Here's the drawing with two shaded views (mm, measured from the low corner). I have some questions. A direction names the side the tool comes from. Round coordinates to 2 decimals unless told otherwise and drop trailing zeros. Write each loop counter-clockwise with the first axis right and the second up, starting at its lowest first coordinate (ties: lowest second). Pieces come first, ordered by that corner, then holes. Notation, with made-up numbers: (55.5, -20) - (67.5, -20) arc R21 ccw to (67.5, 2) - close; hole circle Ø2 at (26.25, 35). An arc over 180 degrees is marked (long way). Return JSON: item names as keys, results as strings. Group by question number.
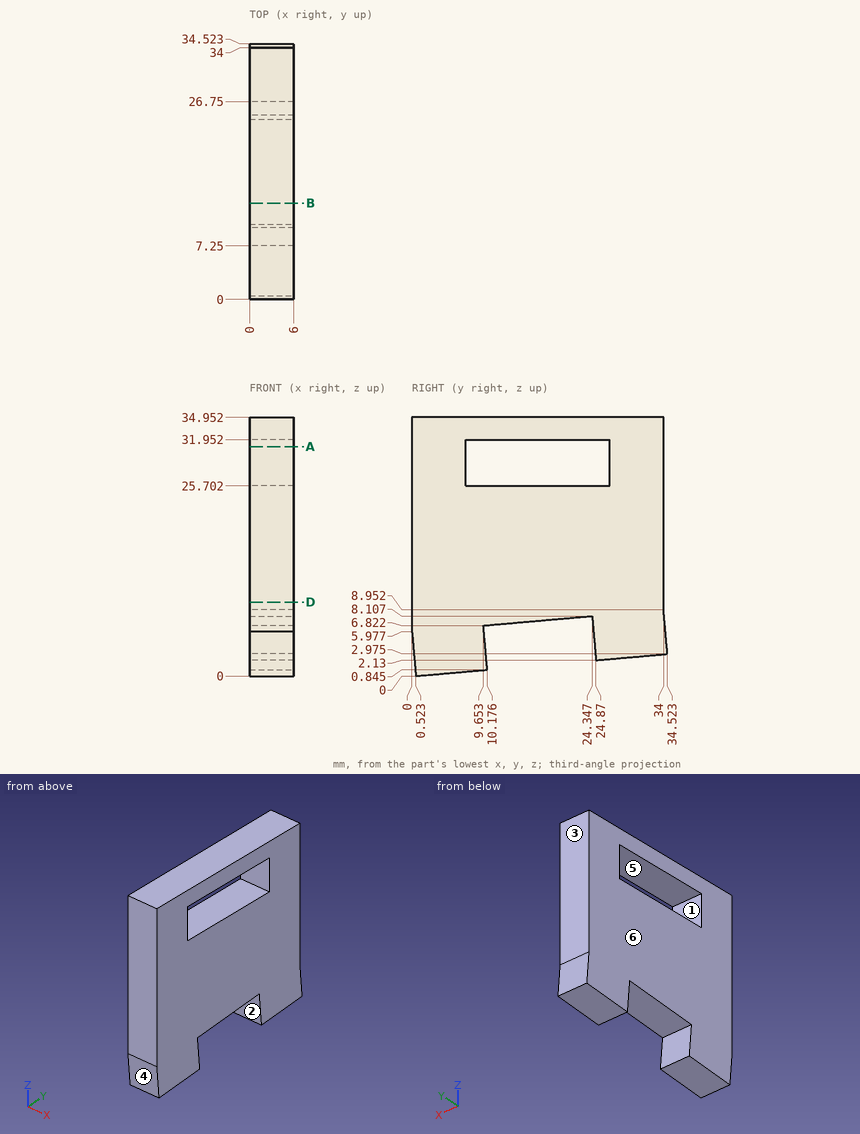
1) Will this pin go through, and if not, where does the flat tip stop? pin 1 Ø3 at (x, z) = (2, 5) entering from +Y.
2) Imagine slicing it at B-B (y = 13). Please give me the cut outline in (x, z) (1 decimal).
3) Imagine slicing it at D-D (z = 10). Please give me the cut outline in (x, y), plus the area to 3 significant figures.
4) If we mould it in two halves opening along Z, with no side actions, what happens to the marked faces 4, 5 and 6? For each: released by +Z, released by -Z, zero draft, split by the parting line, or undercut.
5) Imagine slicing it at A-A (z = 31). Please give me the cut outline in (x, y).
6) For the marked faces 1, 2 and 3, which set-ups out of +Z, -Z, +X, -X, +Y, -Y let a thin tool reach every point of the face, with its end or its side?
7) I need wall thicknesses on line 1 along Y through (x, z) = (1.2, 31); line 2 along Y through (x, z) = (2.9, 16.5); line 3 along Y through (x, z) = (0.8, 5.5) (1 decimal). Which ranges of each line are inside material? Lowest first, please.
Results found:
{
 "1": {"pin 1": "stops at y = 34.48"},
 "2": {"outline": "(0, 7.1) - (6, 7.1) - (6, 25.7) - (0, 25.7) - close; (0, 32) - (6, 32) - (6, 35) - (0, 35) - close"},
 "3": {"outline": "(0, 0) - (6, 0) - (6, 34) - (0, 34) - close", "area": "204 mm²"},
 "4": {"face 4": "released by -Z", "face 5": "undercut", "face 6": "zero draft"},
 "5": {"outline": "(0, 0) - (6, 0) - (6, 7.25) - (0, 7.25) - close; (0, 26.75) - (6, 26.75) - (6, 34) - (0, 34) - close"},
 "6": {"face 1": "+X, -X", "face 2": "-Z, +X, -X", "face 3": "+Z, +X, -X, +Y"},
 "7": {"line 1": "y = 0 to 7.25, 26.75 to 34", "line 2": "y = 0 to 34", "line 3": "y = 0 to 9.8, 24.6 to 34.3"}
}
